Source: CAD feature listing. Evaluate the final solid. Frame: model axes, mm. Face numbers are marked on the shaded views. A direction names the side the tool comes from. Give positions to 0.01 mm unless a question says otherwise; leave off trailing zeros. Order: outer loops, then holes, each group sorted by start corner. A loop starts at its lowest first (then second) coordinate and runs counter-clockwise, first axis right, second up.
1) Material intervals for line 1 (Y direction, x = -9.5, z = 4.5); line 2 (X direction, y = 3.5, z = 1); line 3 (X direction, y = -5.5, z = 1.25), sorted ascending.
2) Section A-A, the plane z = 0.5. Give the number of separate pieces and of enclosed holes in the cut face, plus the area to 3 significant figures.
3) First-contact query: P1, Ø4.5, axis at x = 0, y = -8, coming from the -Z side; P2, Ø3, axis at x = -8, y = 8, coming from the +Z side; P3, Ø4, axis at x = 8.5, y = 0, coming from the -Z side. Flat tips, straight axial feed; report the tip coordinate or a pass-through.
4) Section B-B, the plane y = 4. Return loops of the section in (x, z).
5) Section C-C, the plane z = 8. Return loops of the section in (x, y), plus the area to 3 significant figures.
6) Draft query along Y for the marked faces 4, 5 and 6. Return one class per face: released by +Y, released by -Y, zero draft, split by the parting line, or undercut.
7) Access query for the marked faces 1, 2 and 3. Directions: +Z, -Z, +X, -X, +Y, -Y. A direction counts if a zero-diameter tool reaches every point of the face in a straight line with its end or side. Return the directions, or none.
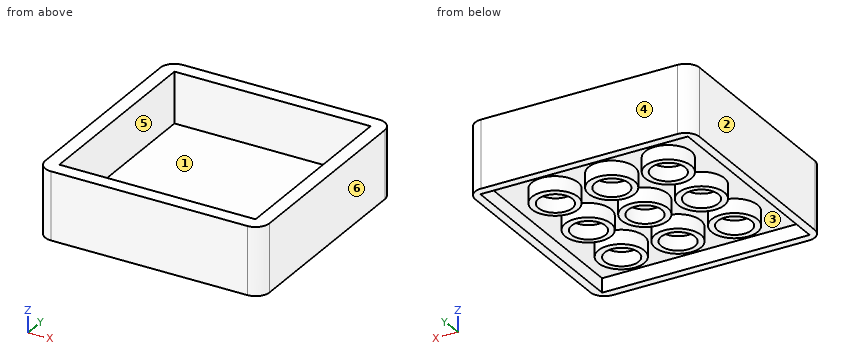
```python
from build123d import *

# Parameters (mm, degrees)
F0_W      = 31.8
F0_H      = 31.8
F1_DEPTH  = 9.6
F2_W      = 29.4
F2_H      = 29.4
F3_DEPTH  = 2
F4_R      = 2
F6_W      = 27.8
F6_H      = 27.8
F7_DEPTH  = 7.2
F8_R      = 3.25685
F10_DEPTH = 2.4
F9_R      = 2.4
F11_DEPTH = 2


with BuildPart() as f1:
    # F0 (on Top) → F1 (new body)
    with BuildSketch(Plane.XY):
        Rectangle(F0_W, F0_H)
    extrude(amount=F1_DEPTH)

    # F2 (on Top) → F3 (cut)
    with BuildSketch(Plane.XY):
        Rectangle(F2_W, F2_H)
    extrude(amount=F3_DEPTH, mode=Mode.SUBTRACT)

    # F4
    f4_edges = [f1.edges().sort_by_distance(p)[0] for p in [
        (-15.9, -15.9, 4.8),
        (-15.9, 15.9, 4.8),
        (15.9, 15.9, 4.8),
        (15.9, -15.9, 4.8),
    ]]
    fillet(f4_edges, radius=F4_R)

    # F6 (on offset) → F7 (cut)
    with BuildSketch(Plane.XY.offset(9.6)):
        Rectangle(F6_W, F6_H)
    extrude(amount=-F7_DEPTH, mode=Mode.SUBTRACT)

    # F8 (on Top) → F10 (join)
    with BuildSketch(Plane.XY):
        with Locations((-8, -8)):
            Circle(F8_R)
        with Locations((-8, 0)):
            Circle(F8_R)
        with Locations((-8, 8)):
            Circle(F8_R)
        with Locations((-0.000151, -7.950921)):
            Circle(F8_R)
        with Locations((-0.000151, 0.049079)):
            Circle(F8_R)
        with Locations((-0.000151, 8.049079)):
            Circle(F8_R)
        with Locations((7.999699, -7.901842)):
            Circle(F8_R)
        with Locations((7.999699, 0.098158)):
            Circle(F8_R)
        with Locations((7.999699, 8.098158)):
            Circle(F8_R)
    extrude(amount=F10_DEPTH)

    # F9 (on Top) → F11 (cut)
    with BuildSketch(Plane.XY):
        with Locations((-8, -8)):
            Circle(F9_R)
        with Locations((-8, 0)):
            Circle(F9_R)
        with Locations((-8, 8)):
            Circle(F9_R)
        with Locations((0, -8)):
            Circle(F9_R)
        Circle(F9_R)
        with Locations((0, 8)):
            Circle(F9_R)
        with Locations((8, -8)):
            Circle(F9_R)
        with Locations((8, 0)):
            Circle(F9_R)
        with Locations((8, 8)):
            Circle(F9_R)
    extrude(amount=F11_DEPTH, mode=Mode.SUBTRACT)


solid = f1.part
```
From the geometry:
1. line 1: y = -15.9 to -13.9, 13.9 to 15.9
1. line 2: x = -15.9 to -14.7, 14.7 to 15.9
1. line 3: x = -15.9 to -14.7, -10.09 to -5.91, -2.14 to 2.14, 5.8 to 10.2, 14.7 to 15.9
2. separate pieces: 10
2. enclosed holes: 10
2. area: 280 mm2
3. P1: stops at z = 2
3. P2: stops at z = 2.4
3. P3: stops at z = 0
4. outline: (-15.9, 0) - (-14.7, 0) - (-14.7, 2) - (14.7, 2) - (14.7, 0) - (15.9, 0) - (15.9, 9.6) - (13.9, 9.6) - (13.9, 2.4) - (-13.9, 2.4) - (-13.9, 9.6) - (-15.9, 9.6) - close
5. outline: (-15.9, -13.9) arc R2 ccw to (-13.9, -15.9) - (13.9, -15.9) arc R2 ccw to (15.9, -13.9) - (15.9, 13.9) arc R2 ccw to (13.9, 15.9) - (-13.9, 15.9) arc R2 ccw to (-15.9, 13.9) - close; hole (-13.9, -13.9) - (13.9, -13.9) - (13.9, 13.9) - (-13.9, 13.9) - close
5. area: 235 mm2
6. face 4: released by +Y
6. face 5: undercut
6. face 6: zero draft
7. face 1: +Z
7. face 2: +Z, -Z, -X, +Y, -Y
7. face 3: -Z
